The listing builds one solid part. Answer for the finished solid, in the listing's coordinates (mm). A direction names the side the tool comes from. Round coordinates to 2 decimals unless told otherwise and drop trailing zeros. Write each loop counter-clockwise with the first axis right and the second up, starting at its lowest first coordinate (ties: lowest second). Pieces come first, ordered by that corner, then holes.
Item 1: Find the intervals of material crossed by probe 1 along X at (y, z) = (19.25, -7.75); probe 2 along X at (y, z) = (17.75, -9.5); probe 3 along Z at (x, y) = (-51, 4.75), in increasing order.
Item 2: A tool of negligible diameter and unlimited length cuts with its end or side. For faces 1 (the face through (-47, 19.5, 0)), 2 (the face through (15.26, -3.451, 10.733)), 3 (the face through (-47, 12, 8.5)), 4 (the face through (0, 1.5, 0)), 5 (the face through (-23, 1, 0)), from which of +Z, -Z, +X, -X, +Y, -Y can it reach the whole face along a straight path? Write none if from no direction.
Item 3: Each of these flat-tipped pins is pushed along its axis until it touches: pin 1 (1.5 mm diameter, centred on x = -24, y = -0.5, fed in from +Z); pin 2 (2.5 mm diameter, centred on x = -22, z = -4.5, fed in from +Y); pin 3 (10 mm diameter, centred on x = -25.5, z = 1.5, fed in from -Y); pin 4 (8 mm diameter, centred on x = -50, y = 11, fed in from +Z). Where does it stop, or does it pass through?
Item 4: Find section C-C on y = 6.75. Give the vertices of the cut face in (x, z).
Item 5: Find section B-B on x = 15. Give the vertices of the cut face in (y, z).
Item 6: For a pull along Z with two mould halves and no side action, classify faces 6 (the face through (-22, 12, -11.5)), 7 (the face through (-24, 19, 0)), 8 (the face through (-70, 19, -1)), 9 (the face through (-47, 11, -8.5)) as +Z half, -Z half, draft (parallel to the pull), parting line (faces both ways), or undercut.
Item 7: Find section D-D on x = -55. Give the vertices of the cut face in (y, z).
Item 8: Find section A-A on z = -2.5. Give the vertices of the cut face in (x, y).
Autodesk Inventor part; units mm, degrees
ref_plane "YZ Plane" through (0, 0, 0) normal (1, 0, 0) x (0, 1, 0)
ref_plane "XZ Plane" through (0, 0, 0) normal (0, 1, 0) x (-1, 0, 0)
ref_plane "XY Plane" through (0, 0, 0) normal (0, 0, 1) x (1, 0, 0)
sketch "Sketch1" plane through (0, 0, 0) normal (0, 1, 0) x (-1, 0, 0)
  line L0 (-20, 12.5) -> (20, 12.5)
  line L1 (20, 12.5) -> (20, -12.5)
  line L2 (20, -12.5) -> (-20, -12.5)
  line L3 (-20, -12.5) -> (-20, 12.5)
  line L4 (-20, 12.5) -> (20, -12.5) construction
  line L5 (20, 12.5) -> (-20, -12.5) construction
  circle A0 centre (-15, 8.75) radius 2
  circle A1 centre (-15, -8.75) radius 2
  point P0 (0, 0)
  dimension "d0" = 40
  dimension "d1" = 25
  dimension "d2" = 4
  dimension "d3" = 4
extrude "Extrusion1" add sketch "Sketch1" along normal blind 1.5 contours L0 L1 L2 L3 | A1
extrude "Extrusion2" add sketch "Sketch1" against normal blind 7 contours A0 | A1
thread "Thread1"
thread "Thread2"
sketch "Sketch2" plane through (15, 0, 8.75) normal (0, 1, 0) x (1, 0, 0)
  circle A0 centre (0, 0) radius 2
  circle A1 centre (0, 0) radius 2
  point P0 (-15, 8.75)
extrude "Extrusion3" add sketch "Sketch2" along normal blind 1.5
sketch "Sketch3" plane through (-20, 0, -12.5) normal (-1, 0, 0) x (0, 0, 1)
  line L0 (0, 0) -> (25, 0)
  line L1 (0, 0) -> (25, 0)
  line L2 (25, 0) -> (25, 22)
  line L3 (25, 22) -> (0, 22)
  line L4 (0, 22) -> (0, 0)
  point P0 (12.5, 0)
  dimension "d14" = 22
extrude "Extrusion4" add sketch "Sketch3" along normal blind 5
sketch "Sketch4" plane through (-20, 22, 12.5) normal (0, 1, 0) x (1, 0, 0)
  line L0 (-4, 24) -> (-1, 24)
  line L1 (-1, 24) -> (-1, 1)
  line L2 (-1, 1) -> (-4, 1)
  line L3 (-4, 1) -> (-4, 24)
  point P0 (20, 12.5)
  dimension "d17" = 3
  dimension "d18" = 23
extrude "Extrusion5" cut sketch "Sketch4" against normal blind 21
sketch "Sketch5" plane through (-25, 0, -12.5) normal (-1, 0, 0) x (0, 0, 1)
  line L0 (20, 18.5) -> (20, 3.5)
  line L1 (20, 3.5) -> (5, 3.5)
  line L2 (5, 3.5) -> (5, 18.5)
  line L3 (5, 18.5) -> (20, 18.5)
  point P0 (12.5, 0)
  dimension "d21" = 15
  dimension "d22" = 15
extrude "Extrusion6" cut sketch "Sketch5" against normal blind 1
sketch "Sketch6" plane through (-21, 22, -11.5) normal (-1, 0, 0) x (0, 0, 1)
  line L0 (0, 0) -> (23, 0)
  line L1 (0, 0) -> (23, 0)
  line L2 (23, 0) -> (23, -2)
  line L3 (23, -2) -> (0, -2)
  line L4 (0, -2) -> (0, 0)
  point P0 (11.5, -22)
  dimension "d26" = 2
extrude "Extrusion7" cut sketch "Sketch6" against normal blind 1
sketch "Sketch7" plane through (-25, 0, -12.5) normal (-1, 0, 0) x (0, 0, 1)
  line L0 (20, 3.5) -> (5, 3.5)
  line L1 (5, 3.5) -> (4, 3.5)
  line L2 (4, 3.5) -> (4, 19.5)
  line L3 (4, 19.5) -> (5, 19.5)
  line L4 (5, 19.5) -> (5, 3.5)
  line L5 (5, 19.5) -> (20, 19.5)
  line L6 (20, 19.5) -> (20, 18.5)
  line L7 (20, 18.5) -> (5, 18.5)
  line L8 (5, 18.5) -> (5, 19.5)
  line L9 (20, 3.5) -> (20, 19.5)
  line L10 (20, 19.5) -> (21, 19.5)
  line L11 (21, 19.5) -> (21, 3.5)
  line L12 (21, 3.5) -> (20, 3.5)
  line L13 (25, 0) -> (25, 22)
  point P0 (12.5, 0)
  dimension "d29" = 1
  dimension "d30" = 16
  dimension "d31" = 15
  dimension "d32" = 1
extrude "Extrusion8" add sketch "Sketch7" along normal blind 1 contours L1 L2 L3 L4
extrude "Extrusion9" add sketch "Sketch7" along normal blind 45 contours L9 L6 L10 L11 L12 | L7 L4 L5 L6
extrude "Extrusion10" add sketch "Sketch7" along normal blind 45 contours L1 L2 L3 L4
properties part number "rgb-holder-group2"
Check values:
1. probe 1: x = -70 to -24, -21 to -20
1. probe 2: x = -25 to -24, -21 to -20
1. probe 3: z = -8.5 to -7.5, 7.5 to 8.5
2. face 1: +Z, -Z, -X, +Y
2. face 2: -Y
2. face 3: +Z, -X, +Y, -Y
2. face 4: +Z, -Z, +X, +Y
2. face 5: +Y
3. pin 1: stops at z = 12.5
3. pin 2: stops at y = 20
3. pin 3: stops at y = 0
3. pin 4: stops at z = 8.5
4. outline: (-70, -8.5) - (-25, -8.5) - (-25, -12.5) - (-20, -12.5) - (-20, 12.5) - (-25, 12.5) - (-25, 8.5) - (-70, 8.5) - (-70, 7.5) - (-24, 7.5) - (-24, 11.5) - (-21, 11.5) - (-21, -11.5) - (-24, -11.5) - (-24, -7.5) - (-70, -7.5) - close
5. outline: (-7, -10.75) - (0, -10.75) - (0, -12.5) - (1.5, -12.5) - (1.5, 12.5) - (0, 12.5) - (0, 10.75) - (-7, 10.75) - (-7, 6.75) - (0, 6.75) - (0, -6.75) - (-7, -6.75) - close
6. face 6: undercut
6. face 7: undercut
6. face 8: draft
6. face 9: -Z half
7. outline: (3.5, -8.5) - (19.5, -8.5) - (19.5, 8.5) - (3.5, 8.5) - (3.5, 7.5) - (18.5, 7.5) - (18.5, -7.5) - (3.5, -7.5) - close
8. outline: (-70, 18.5) - (-24, 18.5) - (-24, 22) - (-25, 22) - (-25, 19.5) - (-70, 19.5) - close; (-25, 0) - (20, 0) - (20, 1.5) - (-20, 1.5) - (-20, 20) - (-21, 20) - (-21, 1) - (-24, 1) - (-24, 3.5) - (-25, 3.5) - close
